Could you check a few things on this drawing? It's one solid part, dimensions in mm from its lowest x, y, z. A direction names the side the tool comes from. Round coordinates to 2 decimals unless told otherwise and drop trailing zeros. Order: outer loops, then holes, each group sorted by start corner. A loop starts at its lowest first (then second) coordinate and runs counter-clockwise, first axis right, second up. Notation, with made-up numbers: M 15.25,-27 L 58.25,-27 A12 ccw 58.25,-23 Z; hole C 72,64 d2. An arc over 180 degrees is marked long. Answer as a JSON object with one key per item and string values. Group by question number.
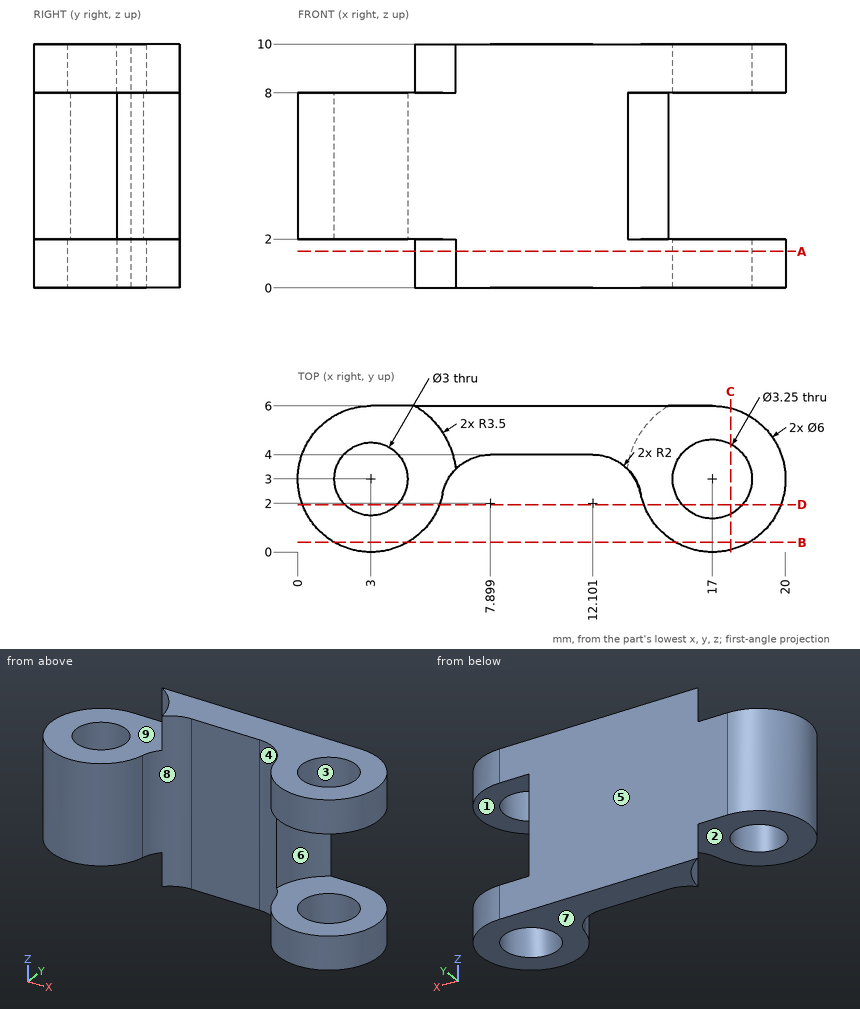
1) We'd pull the mould along Z, two halves only. Please class the marked faces 6, 7, 8 and 9: +Z half, -Z half, draft (parallel to the pull), parting line (faces both ways), or undercut.
2) If we section it at B-B on y = 0.4: Write out the boundary of the cut face in (x, z), plus the area to 3 significant figures.
3) For pin 1 (1.8 mm diameter, centred on x = 2, y = 3, fed in from -Z); pin 2 (2.5 mm diameter, centred on x = 17, y = 3, fed in from -Z); pin 3 (1 mm diameter, centred on x = 12.5, z = 4, fed in from -Y); pin 4 (2 mm diameter, centred on x = 10.5, z = 5.5, fed in from -Y), each with a flat end and sliding along its axis, tell me the tip position at first contact or that it passes through.
4) If we section it at D-D on y = 1.95: Write out the boundary of the cut face in (x, z).
5) I need wall thicknesses on line 1 along Z through (x, y) = (15, 4.65); line 2 along Y through (x, z) = (3, 3.5); line 3 along Z through (x, y) = (6.25, 3.85). Which ranges of each line are inside material? Lowest first, please.
6) Which directions (+Z, -Z, +X, -X, +Y, -Y) give clear straight access to the entire face, cutting with the end or side of a thin tool? Please do the marked faces 1, 2, 3, 4 and 5.
7) If we section it at C-C on x = 17.75: Write out the boundary of the cut face in (y, z).
8) If we section it at A-A on z = 1.5: Write out the boundary of the cut face in (x, y) (3 decimals), plus the area to 3 significant figures.
Findings:
{
 "1": {"face 6": "undercut", "face 7": "-Z half", "face 8": "draft", "face 9": "+Z half"},
 "2": {"outline": "M 1.5,2 L 4.5,2 L 4.5,8 L 1.5,8 Z; M 15.5,0 L 18.5,0 L 18.5,2 L 15.5,2 Z; M 15.5,8 L 18.5,8 L 18.5,10 L 15.5,10 Z", "area": "29.9 mm^2"},
 "3": {"pin 1": "stops at z = 2", "pin 2": "passes through", "pin 3": "stops at y = 3.79", "pin 4": "stops at y = 4"},
 "4": {"outline": "M 0.19,2 L 1.93,2 L 1.93,8 L 0.19,8 Z; M 4.07,2 L 5.81,2 L 5.81,8 L 4.07,8 Z; M 14.19,0 L 15.76,0 L 15.76,2 L 14.19,2 Z; M 14.19,8 L 15.76,8 L 15.76,10 L 14.19,10 Z; M 18.24,0 L 19.81,0 L 19.81,2 L 18.24,2 Z; M 18.24,8 L 19.81,8 L 19.81,10 L 18.24,10 Z"},
 "5": {"line 1": "z = 0 to 2, 8 to 10", "line 2": "y = 0 to 1.5, 4.5 to 6", "line 3": "z = 2 to 8"},
 "6": {"face 1": "+X, -Y", "face 2": "-Z, -X, -Y", "face 3": "+Z, -Z", "face 4": "+Z, -Z, -Y", "face 5": "+Z, -Z, +X, -X, +Y"},
 "7": {"outline": "M 0.1,0 L 1.56,0 L 1.56,2 L 0.1,2 Z; M 0.1,8 L 1.56,8 L 1.56,10 L 0.1,10 Z; M 4.44,0 L 5.9,0 L 5.9,2 L 4.44,2 Z; M 4.44,8 L 5.9,8 L 5.9,10 L 4.44,10 Z"},
 "8": {"outline": "M 4.803,6 A3.5 cw 6.476,3.406 A2 cw 7.899,4 L 12.101,4 A2 cw 14.061,2.4 A3 ccw long 17,6 Z; hole C 17,3 d3.25", "area": "39.3 mm^2"}
}
